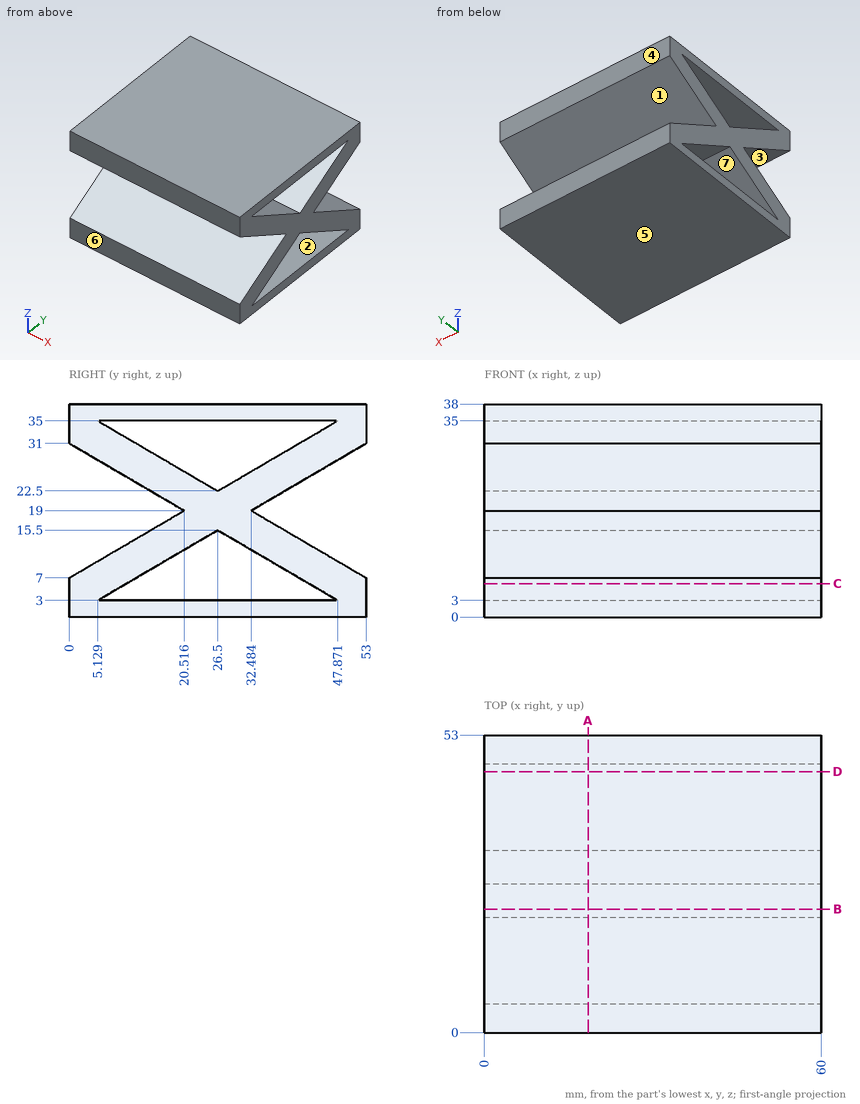
Study the drawing (mm; zero at the part's minimum x, y, z) and answer. A direction names the side the tool comes from. Round coordinates to 2 decimals unless told otherwise and drop trailing zeros. Order: outer loops, then holes, each group sorted by start corner. A loop starts at its lowest first (then second) coordinate and runs counter-clockwise, first axis right, second up. Notation, with made-up numbers: (38, -2) -> (87, -2) arc R22 cw to (87, 5) -> close; hole circle Ø7 at (66, -31). An arc over 180 degrees is marked (long way). Answer as CSV lines item,"result". Start each with the question number.
(1) A tool of negligible diameter and unlimited length cuts with its end or side. For the marked faces 1, 2 and 3, from which of +Z, -Z, +X, -X, +Y, -Y can it reach the whole face along a straight path? Write none if from no direction.
(2) A flat-ended cylindrical pin translates along its axis: pin 1 Ø5 at (x, z) = (46.5, 15.5) entering from -Y. Find the tip coordinate at first contact, or state that the pin passes through.
(3) The part is cut by section C-C (z = 6). Determine the outline of the cut face in (x, y), then the cut area to 3 significant figures.
(4) The part is cut by section B-B (y = 22). Determine the outline of the cut face in (x, z), then the cut area to 3 significant figures.
(5) The part is cut by section A-A (x = 18.5). Determine the outline of the cut face in (y, z).
(6) For a pull along Y with two mould halves and no side action, classify the marked faces 4, 5, 6 and 7 as +Y half, -Y half, draft (parallel to the pull), parting line (faces both ways), or undercut.
(7) Find the intervals of material crossed by probe 1 along Z at (x, y) = (8, 12); probe 2 along Z at (x, y) = (13.5, 8); probe 3 along Z at (x, y) = (25.5, 24.5), in increasing order. Write a range as from..to.
(8) The part is cut by section D-D (y = 46.5). Determine the outline of the cut face in (x, z).
Evaluation:
1,face 1,"+X, -X, +Y"
1,face 2,"+X, -X"
1,face 3,"+X, -X, -Y"
2,pin 1,"y = 10.26"
3,outline,"(0, 0) -> (60, 0) -> (60, 10.26) -> (0, 10.26) -> close; (0, 42.74) -> (60, 42.74) -> (60, 53) -> (0, 53) -> close"
3,area,"1,230 mm²"
4,outline,"(0, 0) -> (60, 0) -> (60, 3) -> (0, 3) -> close; (0, 12.87) -> (60, 12.87) -> (60, 25.13) -> (0, 25.13) -> close; (0, 35) -> (60, 35) -> (60, 38) -> (0, 38) -> close"
4,area,"1,100 mm²"
5,outline,"(0, 0) -> (53, 0) -> (53, 7) -> (32.48, 19) -> (53, 31) -> (53, 38) -> (0, 38) -> (0, 31) -> (20.52, 19) -> (0, 7) -> close; hole (5.13, 3) -> (47.87, 3) -> (26.5, 15.5) -> close; hole (5.13, 35) -> (26.5, 22.5) -> (47.87, 35) -> close"
6,face 4,"+Y half"
6,face 5,"draft"
6,face 6,"-Y half"
6,face 7,"undercut"
7,probe 1,"0..3, 7.02..14.02, 23.98..30.98, 35..38"
7,probe 2,"0..3, 4.68..11.68, 26.32..33.32, 35..38"
7,probe 3,"0..3, 14.33..23.67, 35..38"
8,outline,"(0, 0) -> (60, 0) -> (60, 3) -> (0, 3) -> close; (0, 3.8) -> (60, 3.8) -> (60, 10.8) -> (0, 10.8) -> close; (0, 27.2) -> (60, 27.2) -> (60, 34.2) -> (0, 34.2) -> close; (0, 35) -> (60, 35) -> (60, 38) -> (0, 38) -> close"
